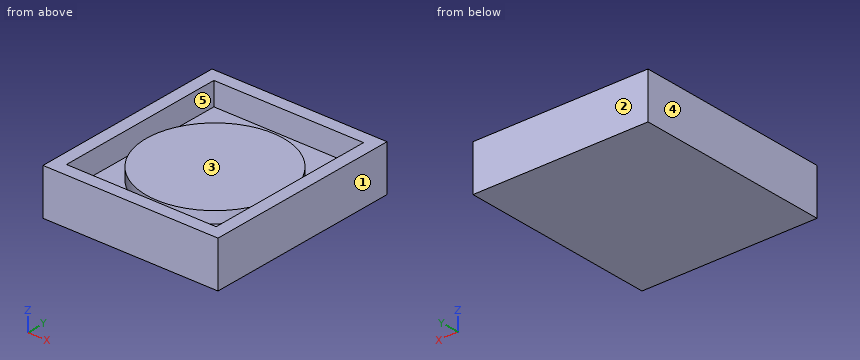
from build123d import *

# Parameters (mm, degrees)
F0_W     = 76
F0_H     = 86
F1_DEPTH = 20
F2_W     = 65
F2_H     = 75
F3_DEPTH = 10
F4_R     = 29.772661
F5_DEPTH = 5


with BuildPart() as f1:
    # F0 (on Top) → F1 (new body)
    with BuildSketch(Plane.XY):
        Rectangle(F0_W, F0_H)
    extrude(amount=F1_DEPTH)

    # F2 (on face) → F3 (cut)
    with BuildSketch(Plane.XY.offset(20)):
        Rectangle(F2_W, F2_H)
    extrude(amount=-F3_DEPTH, mode=Mode.SUBTRACT)

    # F4 (on face) → F5 (join)
    with BuildSketch(Plane.XY.offset(10)):
        Circle(F4_R)
    extrude(amount=F5_DEPTH)


solid = f1.part
Model file for the job. Use its own axes, mm. Face numbers are marked on the shaded views. A direction names the side the tool comes from. Give positions to 0.01 mm unless a question says otherwise; leave off trailing zeros. Loops run counter-clockwise (first coordinate to the right, second up) from the corner with the lowest first, then second, coordinate; pieces in that order, holes last. Notation, with made-up numbers: (44, 22.5) - (56, 22.5) arc R7 ccw to (56, 34.5) - close; hole circle Ø9 at (-20.75, -38). An arc over 180 degrees is marked (long way). Use one line per item in the form item = value.
(1) Cut at D-D (z = 18.5). Give the cut face in (x, y).
Determined:
outline = (-38, -43) - (38, -43) - (38, 43) - (-38, 43) - close; hole (-32.5, -37.5) - (32.5, -37.5) - (32.5, 37.5) - (-32.5, 37.5) - close
(2) Cut at C-C (x = 0). Give the cut face in (y, z), then the cut area to 3 significant figures.
Determined:
outline = (-43, 0) - (43, 0) - (43, 20) - (37.5, 20) - (37.5, 10) - (29.77, 10) - (29.77, 15) - (-29.77, 15) - (-29.77, 10) - (-37.5, 10) - (-37.5, 20) - (-43, 20) - close
area = 1,270 mm^2
(3) 3-axis set-ups, long thin cutter, end or side, ignore diameter. For the marked faces 4 and 5: which of +Z, -Z, +X, -X, +Y, -Y reach the whole face in a straight line?
Determined:
face_4 = +Z, -Z, -X, +Y, -Y
face_5 = +Z
(4) Drill centre lines: L1, parallel to Y at x = 0.5, z = 10.5; L2, parallel to Y at x = -8, z = 12; L3, parallel to Y at x = 26, z = 15.25. Where is each one in solid material? Low to high.
Determined:
L1 = -43 to -37.5, -29.77 to 29.77, 37.5 to 43
L2 = -43 to -37.5, -28.68 to 28.68, 37.5 to 43
L3 = -43 to -37.5, 37.5 to 43
(5) Cut at A-A (z = 12.5). Give the cut face in (x, y).
Determined:
outline = (-38, -43) - (38, -43) - (38, 43) - (-38, 43) - close; circle Ø59.55 at (0, 0); hole (-32.5, -37.5) - (32.5, -37.5) - (32.5, 37.5) - (-32.5, 37.5) - close
(6) Cut at B-B (y = -34.5). Give the cut face in (x, z), then the cut area to 3 significant figures.
Determined:
outline = (-38, 0) - (38, 0) - (38, 20) - (32.5, 20) - (32.5, 10) - (-32.5, 10) - (-32.5, 20) - (-38, 20) - close
area = 870 mm^2
(7) Pull direction Y, two halves, no side cores. Call the marked faces 1, 2 and 3: pulls with the +Y half, pulls with the -Y half, needs draft (parallel to the pull), parting line crosses it, or undercut.
Determined:
face_1 = needs draft
face_2 = pulls with the +Y half
face_3 = undercut
